Model file for the job. Use its own axes, mm. A direction names the side the tool comes from. Give positions to 0.01 mm unless a question says otherwise; leave off trailing zeros. Order: outer loops, then holes, each group sorted by start corner. A loop starts at its lowest first (then second) coordinate and runs counter-clockwise, first axis right, second up. Notation, with made-up numbers: (-16.75, 20.25) -> (-11.75, 20.25) arc R36 cw to (-11.75, 57.25) -> close; hole circle Ø5 at (79, 37). An arc over 180 degrees is marked (long way). Use CSV: the item, a comma, the result in double quotes. Start each with the question number.
1. 3-axis set-ups, long thin cutter, end or side, ignore diameter. For faces 4 (the flat face through (0, 0, -6)), 5 (the cylindrical face through (-0.54, 10.99, 9.94)), 6 (the cylindrical face through (13, 5, 0)), 7 (the flat face through (0, 5, 0)), 8 (the flat face through (0, 12, 7)): which of +Z, -Z, +X, -X, +Y, -Y reach the whole face in a straight line?
2. Drop flat-ended pins along their axis: pin 1 (8 mm diameter, centred on x = 4.5, z = -5.5, fed in from +Y); pin 2 (6 mm diameter, centred on y = 6.5, z = 5.5, fed in from -X). Give the stop position or say it passes through.
3. Cut at A-A on y = 5.75. List the corners of the cut face in (x, z), then the cut area to 3 significant figures.
4. Cut at C-C on y = 1. List the corners of the cut face in (x, z), then the cut area to 3 significant figures.
5. Wall check: line 1 (Z direction, x = 0, y = 1.6); line 2 (Y direction, x = -2.5, z = -8.5); line 3 (X direction, y = 8.75, z = 0.25). Give the ranges that are in metal, low to high. Write a range as from..to.
6. Cut at B-B on x = 0. List the corners of the cut face in (y, z), then the cut area to 3 significant figures.
7. Cut at D-D on y = 8. List the corners of the cut face in (x, z), then the cut area to 3 significant figures.
8. Pull direction X, two halves, no side cores. Call faces 1 (the cylindrical face through (-7.91, 8.732, 10.316)), 2 (the cylindrical face through (-1.08, 2.46, -4.88)), 3 (the flat face through (0, 10, 0)): released by +X, released by -X, zero draft, split by the parting line, or undercut.
```python
from build123d import *

# Parameters (mm, degrees)
SKETCH1_R           = 10
BOSS_EXTRUDE1_DEPTH = 10
SKETCH3_R           = 5
CUT_EXTRUDE1_DEPTH  = 5
SKETCH4_R           = 2.5
BOSS_EXTRUDE2_DEPTH = 2
SKETCH5_R           = 1.25
BOSS_EXTRUDE3_DEPTH = 10


with BuildPart() as part:
    # Sketch1 → Boss-Extrude1 (new body)
    with BuildSketch(Plane(origin=(0, 0, 0), x_dir=(1, 0, 0), z_dir=(0, 1, 0))):
        Circle(SKETCH1_R)
    extrude(amount=BOSS_EXTRUDE1_DEPTH)

    # Sketch2 → Revolve1 (revolve)
    with BuildSketch(Plane(origin=(0, 0, 0), x_dir=(0, 0, -1), z_dir=(1, 0, 0))):
        with BuildLine():
            Line((10, 10), (13, 10))
            Line((13, 10), (13, 7.5))
            Line((13, 7.5), (10.60943551, 6.073395143))
            ThreePointArc((10.60943551, 6.073395143), (10, 5), (10.60943551, 3.926604857))
            Line((10.60943551, 3.926604857), (13, 2.5))
            Line((13, 2.5), (13, 0))
            Line((13, 0), (10, 0))
            Line((10, 0), (9.25, 0))
            Line((9.25, 0), (9.25, 10))
            Line((9.25, 10), (10, 10))
        make_face()
    revolve(axis=Axis((0, 10, 0), (0, -1, 0)))

    # Sketch3 → Cut-Extrude1 (cut)
    with BuildSketch(Plane.XZ):
        Circle(SKETCH3_R)
    extrude(amount=-CUT_EXTRUDE1_DEPTH, mode=Mode.SUBTRACT)

    # Sketch4 → Boss-Extrude2 (add)
    with BuildSketch(Plane(origin=(0, 10, 0), x_dir=(1, 0, 0), z_dir=(0, 1, 0))):
        with Locations((0, -7.5)):
            Circle(SKETCH4_R)
    extrude(amount=BOSS_EXTRUDE2_DEPTH)

    # Sketch5 → Boss-Extrude3 (add)
    with BuildSketch(Plane(origin=(0, 10, 0), x_dir=(1, 0, 0), z_dir=(0, 1, 0))):
        with Locations((11.75, 0)):
            Circle(SKETCH5_R)
    extrude(amount=-BOSS_EXTRUDE3_DEPTH)


solid = part.part
```
Verdict:
1,face 4,"+Z, -Z, +X, -X, -Y"
1,face 5,"+Y"
1,face 6,"none"
1,face 7,"-Y"
1,face 8,"+Z, -Z, +X, -X, +Y"
2,pin 1,"y = 10"
2,pin 2,"x = -12.72"
3,outline,"circle Ø20.5 at (0, 0); circle Ø2.5 at (11.75, 0)"
3,area,"335 mm^2"
4,outline,"circle Ø26 at (0, 0); hole circle Ø10 at (0, 0)"
4,area,"452 mm^2"
5,line 1,"-13..-5, 5..13"
5,line 2,"0..10"
5,line 3,"-13..13"
6,outline,"(0, -13) -> (2.5, -13) -> (3.93, -10.61) arc R1.25 cw to (6.07, -10.61) -> (7.5, -13) -> (10, -13) -> (10, 5) -> (12, 5) -> (12, 10) -> (10, 10) -> (10, 13) -> (7.5, 13) -> (6.07, 10.61) arc R1.25 cw to (3.93, 10.61) -> (2.5, 13) -> (0, 13) -> (0, 5) -> (5, 5) -> (5, -5) -> (0, -5) -> close"
6,area,"201 mm^2"
7,outline,"circle Ø26 at (0, 0)"
7,area,"531 mm^2"
8,face 1,"split by the parting line"
8,face 2,"undercut"
8,face 3,"zero draft"
